```python
from build123d import *

# Parameters (mm, degrees)
BOSS_EXTRUDE1_DEPTH = 3
BOSS_EXTRUDE2_DEPTH = 20
SKETCH3_R           = 6
CUT_EXTRUDE1_DEPTH  = 58


with BuildPart() as part:
    # Sketch1 → Boss-Extrude1 (new body)
    with BuildSketch(Plane.XY):
        with BuildLine():
            ThreePointArc((12.275451386, 39.110148544), (12.067880772, 33.648168724), (13.127719813, 28.28598164))
            ThreePointArc((13.127719813, 28.28598164), (-5.7809e-05, 26.00056132), (-13.127971261, 28.285201272))
            ThreePointArc((-13.127971261, 28.285201272), (-12.06796259, 33.647129894), (-12.275256819, 39.10889939))
            ThreePointArc((-12.275256819, 39.10889939), (0.000238569, 36.332719941), (12.275451386, 39.110148544))
        make_face()
    extrude(amount=BOSS_EXTRUDE1_DEPTH)

    # Sketch2 → Boss-Extrude2 (add)
    with BuildSketch(Plane(origin=(0, 0, 0), x_dir=(-1, 0, 0), z_dir=(0, 0, -1))):
        with BuildLine():
            ThreePointArc((-0.000238569, 33.482719941), (6.116423648, 34.084515432), (11.998357864, 35.867368305))
            ThreePointArc((11.998357864, 35.867368305), (12.080645356, 37.492931332), (12.275256819, 39.10889939))
            ThreePointArc((12.275256819, 39.10889939), (-0.000238569, 36.332719941), (-12.275451386, 39.110148544))
            ThreePointArc((-12.275451386, 39.110148544), (-12.080742195, 37.494064654), (-11.998373995, 35.868378864))
            ThreePointArc((-11.998373995, 35.868378864), (-6.116717522, 34.085055957), (-0.000238569, 33.482719941))
        make_face()
        with BuildLine():
            ThreePointArc((-13.127719813, 28.28598164), (5.7809e-05, 26.00056132), (13.127971261, 28.285201272))
            ThreePointArc((13.127971261, 28.285201272), (12.730383089, 29.661389101), (12.417381714, 31.059244398))
            ThreePointArc((12.417381714, 31.059244398), (5.905e-06, 28.850561321), (-12.417221823, 31.060076762))
            ThreePointArc((-12.417221823, 31.060076762), (-12.730176217, 29.662196758), (-13.127719813, 28.28598164))
        make_face()
    extrude(amount=BOSS_EXTRUDE2_DEPTH)

    # Sketch3 → Cut-Extrude1 (cut)
    with BuildSketch(Plane(origin=(0, 0, 0), x_dir=(1, 0, 0), z_dir=(0, 1, 0))):
        with Locations((9.7284e-05, 7)):
            Circle(SKETCH3_R)
    extrude(amount=CUT_EXTRUDE1_DEPTH, mode=Mode.SUBTRACT)


solid = part.part
```
Build history of the part. All positions in model axes, mm. A direction names the side the tool comes from. Give positions to 0.01 mm unless a question says otherwise; leave off trailing zeros. Order: outer loops, then holes, each group sorted by start corner. A loop starts at its lowest first (then second) coordinate and runs counter-clockwise, first axis right, second up. Notation, with made-up numbers: M 24.5,88.25 L 35.5,88.25 A27 cw 35.5,109.25 Z; hole C 82,57 d4. An arc over 180 degrees is marked long. Write item = value, one per line. Start each with the question number.
(1) Two-plate mould, pull along X, no slides. Class faces 1 (the flat face through (0, 36, -20)), 2 (the cylindrical face through (0, 26, -14)), 3 (the cylindrical face through (5.723, 35.203, -8.802)): released by +X, released by -X, zero draft, split by the parting line, or undercut.
(2) Slice it at B-B on y = 35.5. Write the cut outline in (x, z), plus the area to 3 significant figures.
(3) Which spindle directions (+Z, -Z, +X, -X, +Y, -Y) get a long thin tool onto all of the face, cutting with end or side? Do faces 4 (the cylindrical face through (-0.177, 36.333, -13.45)), 5 (the flat face through (0, 32, 0)). Say none if no direction does.
(4) Pin check, flat tips, straight feed: pin 1 Ø5.5 at (x, y) = (2.5, 31) entering from -Z; pin 2 Ø10 at (x, z) = (-3.5, -11) entering from +Y. Stop position of each tip, or through.
(5) Probe L1, parallel to Z at x = -3.5, y = 36; L2, parallel to Y at x = 9.25, z = -16.5; L3, parallel to Y at x = 4, z = -0.25. List the from-to ranges inside material, lowest first. Write a range as [from, to].
(6) Slice it at D-D on x = 4.5. Write the cut outline in (y, z), plus the area to 3 significant figures.
(7) Slice it at C-C on z = -4.75. Write the cut outline in (x, y).
(8) Slice it at A-A on z = -15.25. Write the cut outline in (x, y), plus the area to 3 significant figures.
Responses:
q1.face_1 = zero draft
q1.face_2 = split by the parting line
q1.face_3 = undercut
q2.outline = M -12,0 L -11.07,0 L -11.07,-20 L 11.07,-20 L 11.07,0 L 12,0 L 12,3 L -12,3 Z; hole C 0,-7 d12
q2.area = 402 mm2
q3.face_4 = +Z, -Z, +Y
q3.face_5 = -Z
q4.pin_1 = -20
q4.pin_2 = 37.63
q5.L1 = [-20, -11.87], [-2.13, 3]
q5.L2 = [27.12, 30.06], [34.88, 37.87]
q5.L3 = [26.21, 29.07], [33.74, 36.61]
q6.outline = M 26.26,-20 L 29.13,-20 L 29.13,-10.97 L 26.26,-10.97 Z; M 26.26,-3.03 L 29.13,-3.03 L 29.13,0 L 33.81,0 L 33.81,-3.03 L 36.69,-3.03 L 36.69,3 L 26.26,3 Z; M 33.81,-20 L 36.69,-20 L 36.69,-10.97 L 33.81,-10.97 Z
q6.area = 101 mm2
q7.outline = M -13.13,28.29 A38.85 ccw -5.56,26.4 L -5.56,29.28 A36 cw -12.42,31.06 A23.5 cw Z; M -12.28,39.11 A23.5 cw -12,35.87 A31.37 ccw -5.56,33.98 L -5.56,36.88 A28.52 cw Z; M 5.56,26.4 A38.85 ccw 13.13,28.29 A23.5 cw 12.42,31.06 A36 cw 5.56,29.28 Z; M 5.56,33.98 A31.37 ccw 12,35.87 A23.5 cw 12.28,39.11 A28.52 cw 5.56,36.88 Z
q8.outline = M -13.13,28.29 A38.85 ccw 13.13,28.29 A23.5 cw 12.42,31.06 A36 cw -12.42,31.06 A23.5 cw Z; M -12.28,39.11 A23.5 cw -12,35.87 A31.37 ccw 12,35.87 A23.5 cw 12.28,39.11 A28.52 cw Z
q8.area = 145 mm2
